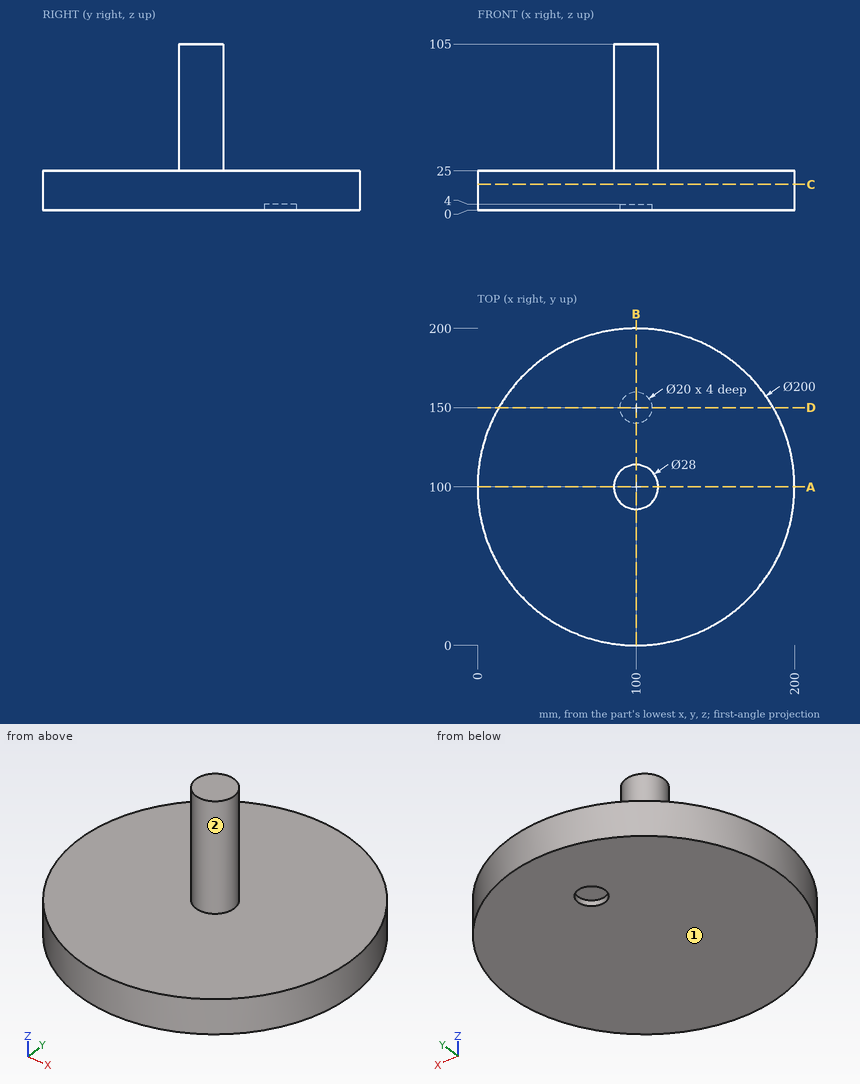
Geometry check sheet. Reference: drawing and pictorial views, mm from the part's lowest x, y, z. A direction names the side the tool comes from. Round coordinates to 2 decimals unless told otherwise and drop trailing zeros. Write each loop counter-clockwise with the first axis right and the second up, starting at its lowest first coordinate (ties: lowest second). Pieces come first, ordered by that corner, then holes. Notation, with made-up numbers: (-31.5, 43.5) -> (8.5, 43.5) arc R20 ccw to (8.5, 57.5) -> close; hole circle Ø2 at (13.5, -15). An arc over 180 degrees is marked (long way). One line per question, with ' | ' between items. Start each with the question number.
1. Set-up check for the marked faces 1 and 2: record each of +Z, -Z, +X, -X, +Y, -Y from which the full face is reachable in a straight line by a thin tool's end or side.
2. Sectioned sample at C-C, the plane z = 16.5. Record the cut outline in (x, y), then the cut area to 3 significant figures.
3. Sectioned sample at A-A, the plane y = 100. Record the cut outline in (x, z).
4. Depth check by flat-ended pin: pin 1 (16 mm diameter, centred on x = 100, y = 150, fed in from -Z); pin 2 (8 mm diameter, centred on x = 23, y = 27.5, fed in from -Z); pin 3 (4 mm diameter, centred on y = 113.5, z = 83, fed in from +X); pin 4 (2 mm diameter, centred on y = 178, z = 20.5, fed in from +X). Enter the tip coordinate at first touch or a pass-through.
5. Sectioned sample at D-D, the plane y = 150. Record the cut outline in (x, z).
6. Scan lines: line 1 along Y through (x, z) = (100, 2.85); line 2 along Z through (x, y) = (75.5, 144); line 3 along X through (y, z) = (159.5, 12.5). Record each from-to range of solid material in increasing order. Write a range as from..to.
7. Sectioned sample at B-B, the plane x = 100. Record the cut outline in (y, z), then the cut area to 3 significant figures.
Taken from the geometry:
1) face 1: -Z, +X, -X, +Y, -Y | face 2: +Z
2) outline: circle Ø200 at (100, 100) | area: 31,400 mm^2
3) outline: (0, 0) -> (200, 0) -> (200, 25) -> (114, 25) -> (114, 105) -> (86, 105) -> (86, 25) -> (0, 25) -> close
4) pin 1: stops at z = 4 | pin 2: passes through | pin 3: stops at x = 107.98 | pin 4: stops at x = 163.8
5) outline: (13.4, 0) -> (90, 0) -> (90, 4) -> (110, 4) -> (110, 0) -> (186.6, 0) -> (186.6, 25) -> (13.4, 25) -> close
6) line 1: y = 0..140, 160..200 | line 2: z = 0..25 | line 3: x = 19.63..180.37
7) outline: (0, 0) -> (140, 0) -> (140, 4) -> (160, 4) -> (160, 0) -> (200, 0) -> (200, 25) -> (114, 25) -> (114, 105) -> (86, 105) -> (86, 25) -> (0, 25) -> close | area: 7,160 mm^2
